```python
from build123d import *

# Parameters (mm, degrees)
SKETCH1_W                = 64
SKETCH1_H                = 75
BOSS_EXTRUDE1_DEPTH      = 9
SKETCH2_W                = 64
SKETCH2_H                = 41
CUT_EXTRUDE1_DEPTH       = 1.5
F_6_0_6_DIAMETER_HOLE1_D = 6


with BuildPart() as part:
    # Sketch1 → Boss-Extrude1 (new body)
    with BuildSketch(Plane(origin=(0, 0, 0), x_dir=(1, 0, 0), z_dir=(0, 1, 0))):
        with Locations((32, 0)):
            Rectangle(SKETCH1_W, SKETCH1_H)
    extrude(amount=BOSS_EXTRUDE1_DEPTH)

    # Sketch2 → Cut-Extrude1 (cut)
    with BuildSketch(Plane.XZ):
        with Locations((32, 0)):
            Rectangle(SKETCH2_W, SKETCH2_H)
    extrude(amount=-CUT_EXTRUDE1_DEPTH, mode=Mode.SUBTRACT)

    # Ø6.0 (6) Diameter Hole1 (through all)
    with Locations(Plane(origin=(0, 9, 0), x_dir=(-1, 0, 0), z_dir=(0, 1, 0))):
        with Locations((-8, 27.5), (-8, -27.5), (-56, -27.5), (-56, 27.5)):
            Hole(F_6_0_6_DIAMETER_HOLE1_D / 2)


solid = part.part
```
Build history of the part. All positions in model axes, mm. A direction names the side the tool comes from. Coordinates: 2 decimals unless noted, no trailing zeros. Order: outer loops, then holes, each group sorted by start corner. A loop starts at its lowest first (then second) coordinate and runs counter-clockwise, first axis right, second up. Notation, with made-up numbers: (4.25, 86) -> (42.25, 86) arc R14 ccw to (42.25, 106) -> close; hole circle Ø7 at (35, -31.75). An arc over 180 degrees is marked (long way). Answer in a Markdown table with one row per item. Add a question column.
Q1. Band-saw the part on A-A, the plane x = 8. List the corners of the cut face in (y, z).
Q2. Wall check: line 1 along Z through (x, y) = (56, 6.25); line 2 along Z through (x, y) = (41, 1); line 3 along Z through (x, y) = (58.5, 5.25). Give the ranges that are in metal, low to high. Write a range as [from, to].
Q3. Band-saw the part on B-B, the plane z = 27.5. List the corners of the cut face in (x, y).
Q4. Band-saw the part on C-C, the plane y = 5. List the corners of the cut face in (x, z), then the cut area to 3 significant figures.
Q5. Band-saw the part on D-D, the plane x = 47. List the corners of the cut face in (y, z), then the cut area to 4 significant figures.
Q6. Mould opens along X. For faces 1 (the face through (10.77, 4.44, -28.65)), 2 (the face through (32, 1, -20.5)), 3 (the face through (64, 4, 1)) say: +X half, -X half, draft (parallel to the pull), parting line (faces both ways), or undercut.
Q7. Which spindle directions (+Z, -Z, +X, -X, +Y, -Y) get a long thin tool onto all of the face, cutting with end or side? Do faces 4 (the face through (10.77, 4.44, 26.35)), 5 (the face through (32, 1, 20.5)). Say none if no direction does.
Answers follow:
| question | item | result |
|---|---|---|
| 1 | outline | (0, -37.5) -> (9, -37.5) -> (9, -30.5) -> (0, -30.5) -> close; (0, -24.5) -> (9, -24.5) -> (9, 24.5) -> (0, 24.5) -> (0, 20.5) -> (1.5, 20.5) -> (1.5, -20.5) -> (0, -20.5) -> close; (0, 30.5) -> (9, 30.5) -> (9, 37.5) -> (0, 37.5) -> close |
| 2 | line 1 | [-37.5, -30.5], [-24.5, 24.5], [30.5, 37.5] |
| 2 | line 2 | [-37.5, -20.5], [20.5, 37.5] |
| 2 | line 3 | [-37.5, -29.16], [-25.84, 25.84], [29.16, 37.5] |
| 3 | outline | (0, 0) -> (5, 0) -> (5, 9) -> (0, 9) -> close; (11, 0) -> (53, 0) -> (53, 9) -> (11, 9) -> close; (59, 0) -> (64, 0) -> (64, 9) -> (59, 9) -> close |
| 4 | outline | (0, -37.5) -> (64, -37.5) -> (64, 37.5) -> (0, 37.5) -> close; hole circle Ø6 at (8, -27.5); hole circle Ø6 at (8, 27.5); hole circle Ø6 at (56, -27.5); hole circle Ø6 at (56, 27.5) |
| 4 | area | 4,690 mm^2 |
| 5 | outline | (0, -37.5) -> (9, -37.5) -> (9, 37.5) -> (0, 37.5) -> (0, 20.5) -> (1.5, 20.5) -> (1.5, -20.5) -> (0, -20.5) -> close |
| 5 | area | 613.5 mm^2 |
| 6 | face 1 | undercut |
| 6 | face 2 | draft |
| 6 | face 3 | +X half |
| 7 | face 4 | +Y, -Y |
| 7 | face 5 | +X, -X, -Y |
